from build123d import *

# Parameters (mm, degrees)
SKETCH1_R                     = 2.286
BOSS_EXTRUDE1_DEPTH           = 1.5875
SKETCH2_R                     = 2.286
CUT_EXTRUDE1_DEPTH            = 118.348360795
SKETCH3_R                     = 1.651
LIPO_HOLDER_HOLES_DEPTH       = 118.348360795
SKETCH4_R                     = 1.651
LORA_THING_PLUS_DEPTH         = 118.348360795
GPS_BREAKOUT_BOARD_DEPTH      = 118.348360795
GPS_BREAKOUT_BOARD_DEPTH_BACK = 118.348360795
SKETCH5_R                     = 1.651
SKETCH6_R                     = 1.651
CUT_EXTRUDE4_DEPTH            = 118.348360795


with BuildPart() as part:
    # Sketch1 → Boss-Extrude1 (new body)
    with BuildSketch(Plane(origin=(0, 0, 0), x_dir=(1, 0, 0), z_dir=(0, 1, 0))):
        Polygon((-25.4, 86.995), (-63.43142, 86.995), (-63.43142, 60.96), (-78.74, 60.96), (-78.74, 25.4), (-71.12, 25.4), (-71.12, -25.4), (-78.74, -25.4), (-78.74, -60.96), (-63.43142, -60.96), (-63.43142, -86.995), (-25.4, -86.995), (-25.4, -79.375), (25.4, -79.375), (25.4, -86.995), (63.43142, -86.995), (63.43142, -60.96), (78.74, -60.96), (78.74, -25.4), (71.12, -25.4), (71.12, 25.4), (78.74, 25.4), (78.74, 60.96), (63.43142, 60.96), (63.43142, 86.995), (25.4, 86.995), (25.4, 79.375), (-25.4, 79.375), align=None)
        with Locations(Location((-57.15, 76.2, 0), (0, 0, 270))):
            Circle(SKETCH1_R, mode=Mode.SUBTRACT)
        with Locations(Location((57.15, 76.2, 0), (0, 0, 270))):
            Circle(SKETCH1_R, mode=Mode.SUBTRACT)
        with Locations(Location((57.15, -76.2, 0), (0, 0, 270))):
            Circle(SKETCH1_R, mode=Mode.SUBTRACT)
        with Locations(Location((-57.15, -76.2, 0), (0, 0, 270))):
            Circle(SKETCH1_R, mode=Mode.SUBTRACT)
    extrude(amount=BOSS_EXTRUDE1_DEPTH)

    # Sketch2 → Cut-Extrude1 (cut, through all)
    with BuildSketch(Plane(origin=(0, 1.5875, 0), x_dir=(1, 0, 0), z_dir=(0, 1, 0))):
        with Locations(Location((-73.66, -30.48, 0), (0, 0, 270))):
            Circle(SKETCH2_R)
        with Locations(Location((-73.66, -55.88, 0), (0, 0, 270))):
            Circle(SKETCH2_R)
        with Locations(Location((73.66, -55.88, 0), (0, 0, 90))):
            Circle(SKETCH2_R)
        with Locations(Location((73.66, -30.48, 0), (0, 0, 90))):
            Circle(SKETCH2_R)
        with Locations(Location((73.66, 30.48, 0), (0, 0, 270))):
            Circle(SKETCH2_R)
        with Locations(Location((73.66, 55.88, 0), (0, 0, 270))):
            Circle(SKETCH2_R)
        with Locations(Location((-73.66, 55.88, 0), (0, 0, 90))):
            Circle(SKETCH2_R)
        with Locations(Location((-73.66, 30.48, 0), (0, 0, 90))):
            Circle(SKETCH2_R)
    extrude(amount=-CUT_EXTRUDE1_DEPTH, mode=Mode.SUBTRACT)

    # Sketch3 → Lipo Holder Holes (cut, through all)
    with BuildSketch(Plane(origin=(0, 1.5875, 0), x_dir=(1, 0, 0), z_dir=(0, 1, 0))):
        with Locations(Location((-50.73142, 41.275, 0), (0, 0, 270))):
            Circle(SKETCH3_R)
        with Locations(Location((10.99058, 41.275, 0), (0, 0, 270))):
            Circle(SKETCH3_R)
        with Locations(Location((10.99058, -13.335, 0), (0, 0, 270))):
            Circle(SKETCH3_R)
        with Locations(Location((-50.73142, -13.335, 0), (0, 0, 270))):
            Circle(SKETCH3_R)
    extrude(amount=-LIPO_HOLDER_HOLES_DEPTH, mode=Mode.SUBTRACT)

    # Sketch4 → LoRa Thing Plus (cut, through all)
    with BuildSketch(Plane(origin=(0, 1.5875, 0), x_dir=(1, 0, 0), z_dir=(0, 1, 0))):
        with Locations(Location((28.77058, 41.275, 0), (0, 0, 270))):
            Circle(SKETCH4_R)
        with Locations(Location((46.55058, 41.275, 0), (0, 0, 270))):
            Circle(SKETCH4_R)
        with Locations(Location((46.55058, -12.065, 0), (0, 0, 270))):
            Circle(SKETCH4_R)
        with Locations(Location((28.77058, -12.065, 0), (0, 0, 270))):
            Circle(SKETCH4_R)
        with Locations(Location((10.99058, 41.275, 0), (0, 0, 270))):
            Circle(SKETCH4_R)
    extrude(amount=-LORA_THING_PLUS_DEPTH, mode=Mode.SUBTRACT)

    # Sketch5 → GPS Breakout Board (cut, two sides: drawn at the far end of the back side and taken through both)
    with BuildSketch(Plane(origin=(0, 1.5875, 0), x_dir=(1, 0, 0), z_dir=(0, 1, 0)).offset(-GPS_BREAKOUT_BOARD_DEPTH_BACK)):
        with Locations(Location((46.55058, -55.245, 0), (0, 0, 270))):
            Circle(SKETCH5_R)
        with Locations(Location((10.99058, -55.245, 0), (0, 0, 270))):
            Circle(SKETCH5_R)
        with Locations(Location((10.99058, -27.305, 0), (0, 0, 270))):
            Circle(SKETCH5_R)
        with Locations(Location((46.55058, -27.305, 0), (0, 0, 270))):
            Circle(SKETCH5_R)
        with Locations(Location((46.55058, -12.065, 0), (0, 0, 270))):
            Circle(SKETCH5_R)
    extrude(amount=GPS_BREAKOUT_BOARD_DEPTH + GPS_BREAKOUT_BOARD_DEPTH_BACK, mode=Mode.SUBTRACT)

    # Sketch6 → Cut-Extrude4 (cut, through all)
    with BuildSketch(Plane(origin=(0, 1.5875, 0), x_dir=(1, 0, 0), z_dir=(0, 1, 0))):
        with Locations(Location((-4.24942, -47.625, 0), (0, 0, 270))):
            Circle(SKETCH6_R)
        with Locations(Location((-24.56942, -47.625, 0), (0, 0, 270))):
            Circle(SKETCH6_R)
        with Locations(Location((-24.56942, -27.305, 0), (0, 0, 270))):
            Circle(SKETCH6_R)
        with Locations(Location((-4.24942, -27.305, 0), (0, 0, 270))):
            Circle(SKETCH6_R)
        with Locations(Location((10.99058, -27.305, 0), (0, 0, 270))):
            Circle(SKETCH6_R)
    extrude(amount=-CUT_EXTRUDE4_DEPTH, mode=Mode.SUBTRACT)


solid = part.part
Work out the finished part from the listing and answer in its coordinate system (mm). Give positions to 0.01 mm unless a question says otherwise; leave off trailing zeros. Loops run counter-clockwise (first coordinate to the right, second up) from the corner with the lowest first, then second, coordinate; pieces in that order, holes last. Notation, with made-up numbers: (52, 85.5) -> (101, 85.5) arc R5 ccw to (101, 93.5) -> close; hole circle Ø5 at (77.25, 16). An arc over 180 degrees is marked (long way). Use a Markdown table: item, result. Add a question column.
1. A flat-ended cylindrical pin translates along its axis: pin 1 Ø0.5 at (y, z) = (1, -73) entering from -X. Find the tip coordinate at first contact, or state that the pin passes through.
2. Section C-C on x = -57.15 is taken. Determine the outline of the cut face in (y, z) (1 decimal).
3. Section A-A on x = 73.66 is taken. Determine the outline of the cut face in (y, z), and give its area (3 significant figures).
4. Section B-B on z = -55.88 is taken. Determine the outline of the cut face in (x, y), and give its area (3 significant figures).
5. Determine the mould class of faces 1 (the flat face through (-1, 1.588, -1)), 2 (the cylindrical face through (-58.03, 0.78, 78.31)) for opening direction X: released by +X, released by -X, zero draft, split by the parting line, or undercut.
6. Section D-D on y = 0.7 is taken. State how many separate pieces and enclosed holes the cut face has, and give its area (3 significant figures).
7. Find the intervals of material crossed by probe 1 along X at (y, z) = (0.85, -76.2); probe 2 along Z at (x, y) = (-51, 0.95) (3 decimals); probe 3 along Z at (x, y) = (-57, 1.35) (3 decimals), in increasing order.
Results below:
| question | item | result |
|---|---|---|
| 1 | pin 1 | stops at x = -63.43 |
| 2 | outline | (0, -87) -> (1.6, -87) -> (1.6, -78.5) -> (0, -78.5) -> close; (0, -73.9) -> (1.6, -73.9) -> (1.6, 73.9) -> (0, 73.9) -> close; (0, 78.5) -> (1.6, 78.5) -> (1.6, 87) -> (0, 87) -> close |
| 3 | outline | (0, -60.96) -> (1.59, -60.96) -> (1.59, -58.17) -> (0, -58.17) -> close; (0, -53.59) -> (1.59, -53.59) -> (1.59, -32.77) -> (0, -32.77) -> close; (0, -28.19) -> (1.59, -28.19) -> (1.59, -25.4) -> (0, -25.4) -> close; (0, 25.4) -> (1.59, 25.4) -> (1.59, 28.19) -> (0, 28.19) -> close; (0, 32.77) -> (1.59, 32.77) -> (1.59, 53.59) -> (0, 53.59) -> close; (0, 58.17) -> (1.59, 58.17) -> (1.59, 60.96) -> (0, 60.96) -> close |
| 3 | area | 83.9 mm^2 |
| 4 | outline | (-78.74, 0) -> (-75.95, 0) -> (-75.95, 1.59) -> (-78.74, 1.59) -> close; (-71.37, 0) -> (71.37, 0) -> (71.37, 1.59) -> (-71.37, 1.59) -> close; (75.95, 0) -> (78.74, 0) -> (78.74, 1.59) -> (75.95, 1.59) -> close |
| 4 | area | 235 mm^2 |
| 5 | face 1 | zero draft |
| 5 | face 2 | undercut |
| 6 | separate pieces | 1 |
| 6 | enclosed holes | 28 |
| 6 | area | 23,900 mm^2 |
| 7 | probe 1 | x = -63.43 to -59.44, -54.86 to 54.86, 59.44 to 63.43 |
| 7 | probe 2 | z = -86.995 to -42.904, -39.646 to 11.706, 14.964 to 86.995 |
| 7 | probe 3 | z = -86.995 to -78.481, -73.919 to 73.919, 78.481 to 86.995 |
